```python
from build123d import *

# Parameters (mm, degrees)
F0_W     = 12.7
F0_H     = 63.5
F1_DEPTH = 63.5
F2_W     = 12.7
F2_H     = 63.5
F3_DEPTH = 63.5
F4_W     = 50.8
F4_H     = 12.7
F5_DEPTH = 50.8
F6_W     = 12.7
F6_H     = 12.365417
F7_DEPTH = 50.8


with BuildPart() as f1:
    # F0 (on Front) → F1 (new body)
    with BuildSketch(Plane.XZ):
        with Locations((6.35, -31.75)):
            Rectangle(F0_W, F0_H)
    extrude(amount=F1_DEPTH)

    # F2 (on Right) → F3 (join)
    with BuildSketch(Plane.YZ):
        with Locations((-6.35, -31.75)):
            Rectangle(F2_W, F2_H)
    extrude(amount=F3_DEPTH)

    # F4 (on Front) → F5 (join)
    with BuildSketch(Plane.XZ):
        with Locations((37.57162, -57.778161)):
            Rectangle(F4_W, F4_H)
    extrude(amount=F5_DEPTH)

    # F6 (on Right) → F7 (join)
    with BuildSketch(Plane.YZ):
        with Locations((-57.15, -57.474271)):
            Rectangle(F6_W, F6_H)
    extrude(amount=F7_DEPTH)


solid = f1.part
```
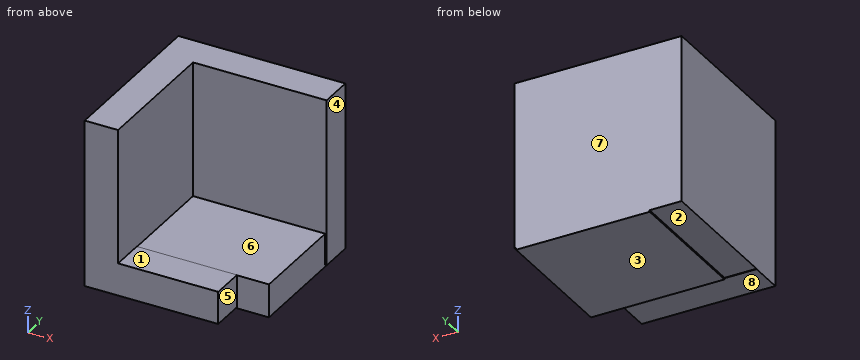
Design review of the part built by this model. Coordinates are the model's own, in mm. Face numbers are marked on the shaded views. A direction names the side the tool comes from. Give positions to 0.01 mm unless a question says otherwise; leave off trailing zeros. Loops run counter-clockwise (first coordinate to the right, second up) from the corner with the lowest first, then second, coordinate; pieces in that order, holes last. Notation, with made-up numbers: M 81,54.25 L 125,54.25 A27 ccw 125,77.25 Z; hole C 9,45 d10. An arc over 180 degrees is marked long. Return JSON: item names as keys, results as strings. Group by question number.
Item 1: We need section B-B (x = 38.5). Give the boundary of the cut face in (y, z), and give its area (3 significant figures).
Item 2: Tool access review of the marked faces 1, 2, 3, 4 and 5: name each direction out of +Z, -Z, +X, -X, +Y, -Y from which nothing blocks a thin tool from reaching the whole face with its end or side.
Item 3: We need section C-C (z = -10.5). Give the boundary of the cut face in (x, y), and give its area (3 significant figures).
Item 4: We need section D-D (x = 59). Give the boundary of the cut face in (y, z).
Item 5: Insertion check: pin 1 Ø6.5 at (y, z) = (-19.5, -57) entering from +X; pin 2 Ø10 at (y, z) = (-56, -56) entering from +X; pin 3 Ø1.5 at (x, z) = (45.5, -31) entering from -Y. Each pin has a flat end and moves straight along its axis. Give the tip position at first contact, or say it passes through.
Item 6: Mouldability with a two-part tool opening along Y and no side actions: class the marked faces 6, 7 and 8 as released by +Y, released by -Y, zero draft, split by the parting line, or undercut.
Item 7: For probe 1 along Y at (x, z) = (45, -31.5); probe 2 along X at (y, z) = (-43.5, -37.5); probe 3 along Z at (x, y) = (54, -36.5), list the stretches that pass through material, from the lowest coordinate up.
Item 8: We need section A-A (y = -14.5). Give the boundary of the cut face in (x, z).
Output:
{
 "1": {"outline": "M -63.5,-63.66 L -50.8,-63.66 L -50.8,-64.13 L 0,-64.13 L 0,0 L -12.7,0 L -12.7,-51.43 L -50.8,-51.43 L -50.8,-51.29 L -63.5,-51.29 Z", "area": "1,460 mm^2"},
 "2": {"face 1": "+Z, +X, -Y", "face 2": "-Z, -X, +Y", "face 3": "-Z, +X, -X, +Y, -Y", "face 4": "+Z, -Z, +X, +Y, -Y", "face 5": "+Z, -Z, +X, -Y"},
 "3": {"outline": "M 0,-63.5 L 12.7,-63.5 L 12.7,-12.7 L 63.5,-12.7 L 63.5,0 L 0,0 Z", "area": "1,450 mm^2"},
 "4": {"outline": "M -50.8,-64.13 L 0,-64.13 L 0,0 L -12.7,0 L -12.7,-51.43 L -50.8,-51.43 Z"},
 "5": {"pin 1": "stops at x = 62.97", "pin 2": "stops at x = 50.8", "pin 3": "stops at y = -12.7"},
 "6": {"face 6": "undercut", "face 7": "released by +Y", "face 8": "zero draft"},
 "7": {"probe 1": "y = -12.7 to 0", "probe 2": "x = 0 to 12.7", "probe 3": "z = -64.13 to -51.43"},
 "8": {"outline": "M 0,-63.5 L 12.17,-63.5 L 12.17,-64.13 L 62.97,-64.13 L 62.97,-51.43 L 12.7,-51.43 L 12.7,0 L 0,0 Z"}
}
